Autodesk Inventor part; units mm, degrees
ref_plane "YZ Plane" through (0, 0, 0) normal (1, 0, 0) x (0, 1, 0)
ref_plane "XZ Plane" through (0, 0, 0) normal (0, 1, 0) x (-1, 0, 0)
ref_plane "XY Plane" through (0, 0, 0) normal (0, 0, 1) x (1, 0, 0)
sketch "Sketch1" plane through (0, 0, 0) normal (0, 1, 0) x (-1, 0, 0)
  line L0 (27.25, 27.25) -> (-27.25, 27.25)
  line L1 (-27.25, 27.25) -> (-27.25, -27.25)
  line L2 (-27.25, -27.25) -> (27.25, -27.25)
  line L3 (27.25, -27.25) -> (27.25, 27.25)
  line L4 (27.25, 27.25) -> (-27.25, -27.25) construction
  line L5 (-27.25, 27.25) -> (27.25, -27.25) construction
  line L6 (21, 21) -> (-21, 21)
  line L7 (-21, 21) -> (-21, -21)
  line L8 (-21, -21) -> (21, -21)
  line L9 (21, -21) -> (21, 21)
  line L10 (21, 21) -> (-21, -21) construction
  line L11 (-21, 21) -> (21, -21) construction
  point P0 (0, 0)
  dimension "d0" = 54.5
  dimension "d1" = 54.5
  dimension "d2" = 42
  dimension "d3" = 42
extrude "Extrusion1" add sketch "Sketch1" along normal blind 6 contours L3 L2 L1 L0 | L9 L8 L7 L6
sketch "Sketch2" plane through (0, 6, 0) normal (0, 1, 0) x (1, 0, 0)
  circle A0 centre (0, 0) radius 25
  dimension "d7" = 50
extrude "Extrusion2" add sketch "Sketch2" along normal blind 2.5
sketch "Sketch3" plane through (0, 0, 0) normal (0, -1, 0) x (1, 0, 0)
  circle A0 centre (0, 0) radius 26
  dimension "d10" = 52
extrude "Extrusion3" add sketch "Sketch3" along normal blind 126
fillet "Fillet1" radius 2.5 1 edges at (-26, -126, 0)
hole "Hole1" at (21, 0, -21) at (21, 0, 21) at (-21, 0, -21) at (-21, 0, 21) direction (0, 1, 0) diameter 4.4 end through all
sketch "Sketch4" plane through (0, 8.5, 0) normal (0, 1, 0) x (1, 0, 0)
  circle A0 centre (0, 0) radius 4
  dimension "d22" = 8
extrude "Extrusion4" add sketch "Sketch4" along normal blind 25
chamfer "Chamfer1" distance 6.5 angle 45 4 edges at (27.25, 3, 27.25) (27.25, 3, -27.25) (-27.25, 3, -27.25) (-27.25, 3, 27.25)
equation "\"d1\" = d0"
equation "\"d3\" = d2"
properties part number "Nanotec-DH052-120E-4N02-Servo"
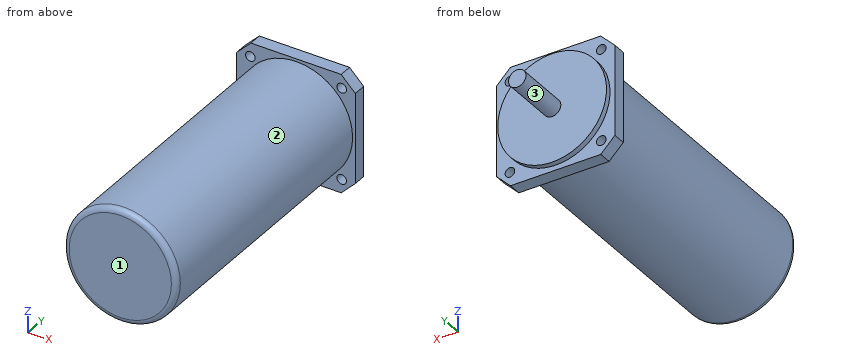
Could you check a few things on this model? Use its own coordinates, in mm. Face numbers are marked on the shaded views. A direction names the side the tool comes from. Give positions to 0.01 mm unless a question says otherwise; leave off trailing zeros. Write each loop counter-clockwise with the first axis right and the second up, starting at its lowest first coordinate (ties: lowest second). Pieces come first, ordered by that corner, then holes. Notation, with made-up numbers: (14.25, 52) - (34.25, 52) arc R26 cw to (34.25, 90) - close; hole circle Ø6 at (58, 15). An arc over 180 degrees is marked (long way). Use CSV: the item, a comma, the result in double quotes. Start each with the question number.
Item 1: For the marked faces 1, 2 and 3, which set-ups out of +Z, -Z, +X, -X, +Y, -Y let a thin tool reach every point of the face, with its end or its side?
Item 2: I want a section at B-B, the plane y = -11. Please give me the cut outline in (x, z), then the cut area to 3 significant figures.
Item 3: I want a section at A-A, the plane z = 0. Please give me the cut outline in (x, y), then the cut area to 3 significant figures.
Item 4: I'm going to push flat-ended pins straight in: pin 1 (5.5 mm diameter, centred on x = -21, z = -21, fed in from -Y); pin 2 (5 mm diameter, centred on x = -7.5, y = -8.5, fed in from +Z); pin 3 (10 mm diameter, centred on x = -8, y = -21.5, fed in from +Z); pin 4 (2.5 mm diameter, centred on x = -21, z = 21, fed in from +Y). Where does each tip first touch, or does it pass through?
Item 5: If I drill on line 1 along X through (y, z) = (2.6, -21); line 2 along Y through (x, z) = (-17, -1.5), over which ranges is the centre line in solid material (lowest first)?
Findings:
1,face 1,"+Z, -Z, +X, -X, -Y"
1,face 2,"-Y"
1,face 3,"+Y"
2,outline,"circle Ø52 at (0, 0)"
2,area,"2,120 mm2"
3,outline,"(-27.25, 0) - (-26, 0) - (-26, -123.5) arc R2.5 ccw to (-23.5, -126) - (23.5, -126) arc R2.5 ccw to (26, -123.5) - (26, 0) - (27.25, 0) - (27.25, 6) - (25, 6) - (25, 8.5) - (4, 8.5) - (4, 33.5) - (-4, 33.5) - (-4, 8.5) - (-25, 8.5) - (-25, 6) - (-27.25, 6) - close"
3,area,"7,200 mm2"
4,pin 1,"stops at y = 0"
4,pin 2,"stops at z = 25.51"
4,pin 3,"stops at z = 25.83"
4,pin 4,"passes through"
5,line 1,"x = -27 to -23.2, -18.8 to 18.8, 23.2 to 27"
5,line 2,"y = -126 to 8.5"
